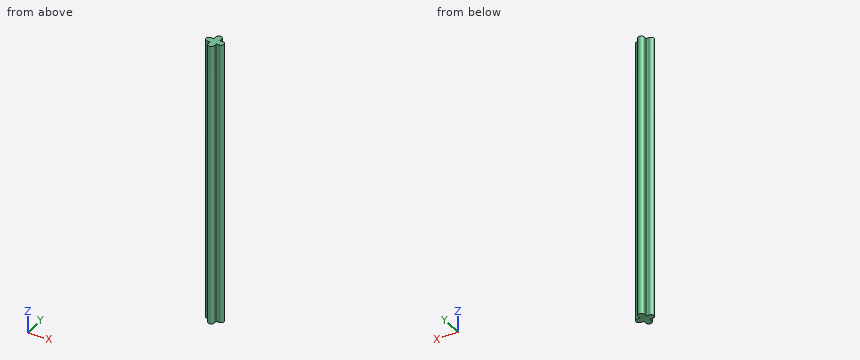
```python
from build123d import *

# Parameters (mm, degrees)
BOSS_EXTRUDE1_DEPTH = 70.866


with BuildPart() as part:
    # Sketch1 → Boss-Extrude1 (new body)
    with BuildSketch(Plane.XY):
        with BuildLine():
            Line((-1.524, 0.762), (1.524, 0.762))
            ThreePointArc((1.524, 0.762), (2.286, 0), (1.524, -0.762))
            Line((1.524, -0.762), (-1.524, -0.762))
            ThreePointArc((-1.524, -0.762), (-2.286, 0), (-1.524, 0.762))
        make_face()
        with BuildLine():
            Line((0.762, 1.524), (0.762, -1.524))
            ThreePointArc((0.762, -1.524), (0, -2.286), (-0.762, -1.524))
            Line((-0.762, -1.524), (-0.762, 1.524))
            ThreePointArc((-0.762, 1.524), (0, 2.286), (0.762, 1.524))
        make_face()
    extrude(amount=BOSS_EXTRUDE1_DEPTH)


solid = part.part
```
For this review, take the finished solid that the model builds, in its own axes (mm). Round coordinates to 2 decimals unless told otherwise and drop trailing zeros. Write each loop counter-clockwise with the first axis right and the second up, starting at its lowest first coordinate (ties: lowest second). Pieces come first, ordered by that corner, then holes. Notation, with made-up numbers: (31, -0.75) -> (65, -0.75) arc R8 cw to (65, 5.25) -> close; hole circle Ø8 at (-32.75, 76). An arc over 180 degrees is marked (long way). Use one line per item in the form item = value.
1) Clearance check with flat-ended pins moving along their axes: pin 1 (2 mm diameter, centred on x = -1.5, z = 62, fed in from +Y); pin 2 (0.8 mm diameter, centred on y = 1, z = 43, fed in from +X); pin 3 (0.6 mm diameter, centred on y = -1.5, z = 24, fed in from -X). State where each tip first meets the part, or that it passes through.
Found:
pin_1 = 2.1
pin_2 = 1.99
pin_3 = -0.76
2) To check wall thickness, follow L1, parallel to X at y = -0.95, z = 62.5; L2, parallel to Y at x = 0.1, z = 17. State the ranges of each line that lie inside material, in increasing order. Write a range as from..to.
Found:
L1 = -0.76..0.76
L2 = -2.28..2.28
3) Take a section at A-A, the plane z = 31.5. Write out the cut boundary in (x, y).
Found:
outline = (-1.52, -0.76) -> (-0.76, -0.76) -> (-0.76, -1.52) arc R0.76 ccw to (0.76, -1.52) -> (0.76, -0.76) -> (1.52, -0.76) arc R0.76 ccw to (1.52, 0.76) -> (0.76, 0.76) -> (0.76, 1.52) arc R0.76 ccw to (-0.76, 1.52) -> (-0.76, 0.76) -> (-1.52, 0.76) arc R0.76 ccw to start
